```python
from build123d import *

# Parameters (mm, degrees)
SKETCH1_W           = 100
SKETCH1_H           = 100
BOSS_EXTRUDE1_DEPTH = 700
SKETCH2_R           = 25
BOSS_EXTRUDE2_DEPTH = 100


with BuildPart() as part:
    # Sketch1 → Boss-Extrude1 (new body)
    with BuildSketch(Plane.XY):
        with Locations((50, 50)):
            Rectangle(SKETCH1_W, SKETCH1_H)
    extrude(amount=BOSS_EXTRUDE1_DEPTH)

    # Sketch2 → Boss-Extrude2 (add)
    with BuildSketch(Plane.XY):
        with Locations((50, 50)):
            Circle(SKETCH2_R)
    extrude(amount=-BOSS_EXTRUDE2_DEPTH)


solid = part.part
```
CAD build for the part. Positions are in the model's coordinates, mm. A direction names the side the tool comes from. Give positions to 0.01 mm unless a question says otherwise; leave off trailing zeros. Order: outer loops, then holes, each group sorted by start corner. A loop starts at its lowest first (then second) coordinate and runs counter-clockwise, first axis right, second up. Notation, with made-up numbers: M -0.75,16.5 L 29.25,16.5 A24 cw 29.25,46.5 Z; hole C 13.5,51.25 d8. An arc over 180 degrees is marked long. Put each result on its own line as item: value. Start each with the question number.
(1) Mould opens along Y. For faces 3 (the flat face through (0, 49, 345)), 4 (the flat face through (49, 100, 345)), 5 (the cylindrical face through (30, 35, -49)) say: +Y half, -Y half, draft (parallel to the pull), parting line (faces both ways), or undercut.
(2) Saw through at A-A, the plane y = 50. Write the cut outline in (x, z).
(3) Which spindle directions (+Z, -Z, +X, -X, +Y, -Y) get a long thin tool onto all of the face, cutting with end or side? Do faces 1 (the flat face through (38, 73, 0)), 2 (the flat face through (50, 50, -100)). Say none if no direction does.
(4) Saw through at C-C, the plane y = 83. Write the cut outline in (x, z).
(5) Drill centre lines: line 1 along Z through (x, y) = (75, 16); line 2 along X through (y, z) = (56.5, -57); line 3 along Y through (x, z) = (34.5, -21.5). Where is each one in solid material? Low to high.
Check result:
1. face 3: draft
1. face 4: +Y half
1. face 5: parting line
2. outline: M 0,0 L 25,0 L 25,-100 L 75,-100 L 75,0 L 100,0 L 100,700 L 0,700 Z
3. face 1: -Z
3. face 2: -Z, +X, -X, +Y, -Y
4. outline: M 0,0 L 100,0 L 100,700 L 0,700 Z
5. line 1: z = 0 to 700
5. line 2: x = 25.86 to 74.14
5. line 3: y = 30.38 to 69.62
